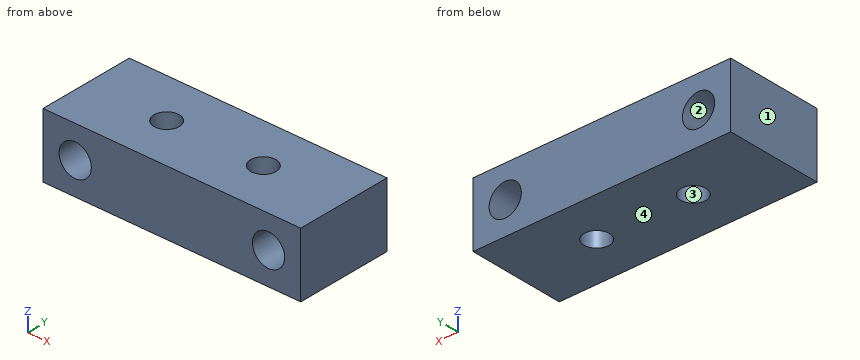
```python
from build123d import *

# Parameters (mm, degrees)
SKETCH1_W           = 50.8
SKETCH1_H           = 19.05
BOSS_EXTRUDE1_DEPTH = 12.7
SKETCH2_R           = 2.5
CUT_EXTRUDE1_DEPTH  = 30.952890094
SKETCH3_R           = 3.175
CUT_EXTRUDE2_DEPTH  = 35.195796525


with BuildPart() as part:
    # Sketch1 → Boss-Extrude1 (new body)
    with BuildSketch(Plane.XY):
        Rectangle(SKETCH1_W, SKETCH1_H)
    extrude(amount=BOSS_EXTRUDE1_DEPTH)

    # Sketch2 → Cut-Extrude1 (cut, through all)
    with BuildSketch(Plane.XY.offset(12.7)):
        with Locations((-9.525, 0)):
            Circle(SKETCH2_R)
        with Locations(Location((9.525, 0, 0), (0, 0, 180))):
            Circle(SKETCH2_R)
    extrude(amount=-CUT_EXTRUDE1_DEPTH, mode=Mode.SUBTRACT)

    # Sketch3 → Cut-Extrude2 (cut, through all)
    with BuildSketch(Plane(origin=(0, 9.525, 0), x_dir=(1, 0, 0), z_dir=(0, 1, 0))):
        with Locations(Location((-19.05, -6.35, 0), (0, 0, 270))):
            Circle(SKETCH3_R)
        with Locations(Location((19.05, -6.35, 0), (0, 0, 270))):
            Circle(SKETCH3_R)
    extrude(amount=-CUT_EXTRUDE2_DEPTH, mode=Mode.SUBTRACT)


solid = part.part
```
For this review, take the finished solid that the model builds, in its own axes (mm). Face numbers are marked on the shaded views. Coordinates: 2 decimals unless noted, no trailing zeros. Loops run counter-clockwise (first coordinate to the right, second up) from the corner with the lowest first, then second, coordinate; pieces in that order, holes last. Notation, with made-up numbers: (84.5, -12.5) - (122.5, -12.5) arc R23 ccw to (122.5, 4.5) - close; hole circle Ø10 at (60, 61). An arc over 180 degrees is marked (long way). Use one line per item in the form item = value. Start each with the question number.
1) Take a section at D-D (y = -7.5). State the section outline as (x, z) points (3 decimals), plus the area to 3 significant figures.
2) For pin 1 (4.5 mm diameter, centred on x = -9.525, y = 0, fed in from +Z), flat-tipped, find the tip position at first contact; note if it passes through.
3) Take a section at A-A (z = 6.35). State the section outline as (x, y) points (3 decimals), plus the area to 3 significant figures.
4) Take a section at C-C (y = 0). State the section outline as (x, z) points (3 decimals).
5) To check wall thickness, follow probe 1 along X at (y, z) = (0.25, 8); probe 2 along X at (y, z) = (-8.25, 4); probe 3 along X at (y, z) = (-0.25, 1.25). State the ranges of each line that lie inside material, in increasing order. Write a range as from..to.
6) Take a section at B-B (x = -19.05). State the section outline as (y, z) points (3 decimals).
7) Draft analysis for pull direction X (two halves, no side actions). For the marked faces 1, 2, 3 and 4, state which applies: released by +X, released by -X, zero draft, split by the parting line, or undercut.
From the geometry:
q1.outline = (-25.4, 0) - (25.4, 0) - (25.4, 12.7) - (-25.4, 12.7) - close; hole circle Ø6.35 at (-19.05, 6.35); hole circle Ø6.35 at (19.05, 6.35)
q1.area = 582 mm2
q2.pin_1 = through
q3.outline = (-25.4, -9.525) - (-22.225, -9.525) - (-22.225, 9.525) - (-25.4, 9.525) - close; (-15.875, -9.525) - (15.875, -9.525) - (15.875, 9.525) - (-15.875, 9.525) - close; (22.225, -9.525) - (25.4, -9.525) - (25.4, 9.525) - (22.225, 9.525) - close; hole circle Ø5 at (-9.525, 0); hole circle Ø5 at (9.525, 0)
q3.area = 687 mm2
q4.outline = (-25.4, 0) - (-12.025, 0) - (-12.025, 12.7) - (-25.4, 12.7) - close; (-7.025, 0) - (7.025, 0) - (7.025, 12.7) - (-7.025, 12.7) - close; (12.025, 0) - (25.4, 0) - (25.4, 12.7) - (12.025, 12.7) - close; hole circle Ø6.35 at (-19.05, 6.35); hole circle Ø6.35 at (19.05, 6.35)
q5.probe_1 = -25.4..-21.76, -16.34..-12.01, -7.04..7.04, 12.01..16.34, 21.76..25.4
q5.probe_2 = -25.4..-21.18, -16.92..16.92, 21.18..25.4
q5.probe_3 = -25.4..-12.01, -7.04..7.04, 12.01..25.4
q6.outline = (-9.525, 0) - (9.525, 0) - (9.525, 3.175) - (-9.525, 3.175) - close; (-9.525, 9.525) - (9.525, 9.525) - (9.525, 12.7) - (-9.525, 12.7) - close
q7.face_1 = released by -X
q7.face_2 = undercut
q7.face_3 = undercut
q7.face_4 = zero draft
